Input: part model. Units: mm. Frame: model coordinates. Face numbers are marked on the shaded views. A direction names the side the tool comes from. Give positions to 0.01 mm unless a question says otherwise; leave off trailing zeros. Write each loop counter-clockwise with the first axis right and the second up, starting at its lowest first coordinate (ties: lowest second). Pieces come first, ordered by that corner, then holes. Notation, with made-up numbers: (27.25, -18) - (56.25, -18) arc R30 ccw to (56.25, 5) - close; hole circle Ø8 at (67.25, 6.5). An arc over 180 degrees is marked (long way). Answer as a JSON object with one key per item and string values. Group by question number.
from build123d import *

# Parameters (mm, degrees)
SKETCH_1_R               = 7
EXTRUDE_1_DEPTH          = 12.4
SKETCH_2_W               = 10.589204791
SKETCH_2_H               = 7.5
EXTRUDE_2_DEPTH          = 2
SKETCH_3_R               = 5
CUT_EXTRUDE_1_DEPTH      = 8
CUT_EXTRUDE_1_DEPTH_BACK = 1.5
SKETCH_4_R               = 3.1
CUT_EXTRUDE_2_DEPTH      = 16


with BuildPart() as part:
    # Эскиз1 → Бобышка-Вытянуть1 (new body)
    with BuildSketch(Plane.XY):
        Circle(SKETCH_1_R)
    extrude(amount=EXTRUDE_1_DEPTH)

    # Эскиз2 → Бобышка-Вытянуть2 (add)
    with BuildSketch(Plane.XY):
        with Locations((-11.205397604, 0)):
            Rectangle(SKETCH_2_W, SKETCH_2_H)
    extrude(amount=EXTRUDE_2_DEPTH)

    # Эскиз3 → Вырез-Вытянуть1 (cut, two sides)
    with BuildSketch(Plane(origin=(0, 0, 0), x_dir=(0, 0, -1), z_dir=(1, 0, 0))) as cut_extrude_1_sk:
        with Locations((-6.2, 0)):
            Circle(SKETCH_3_R)
    extrude(amount=CUT_EXTRUDE_1_DEPTH, mode=Mode.SUBTRACT)
    extrude(cut_extrude_1_sk.sketch, amount=-CUT_EXTRUDE_1_DEPTH_BACK, mode=Mode.SUBTRACT)

    # Эскиз4 → Вырез-Вытянуть2 (cut, through all)
    with BuildSketch(Plane(origin=(-1.5, 0, 0), x_dir=(0, 0, -1), z_dir=(1, 0, 0))):
        with Locations((-6.2, 0)):
            Circle(SKETCH_4_R)
    extrude(amount=-CUT_EXTRUDE_2_DEPTH, mode=Mode.SUBTRACT)


solid = part.part
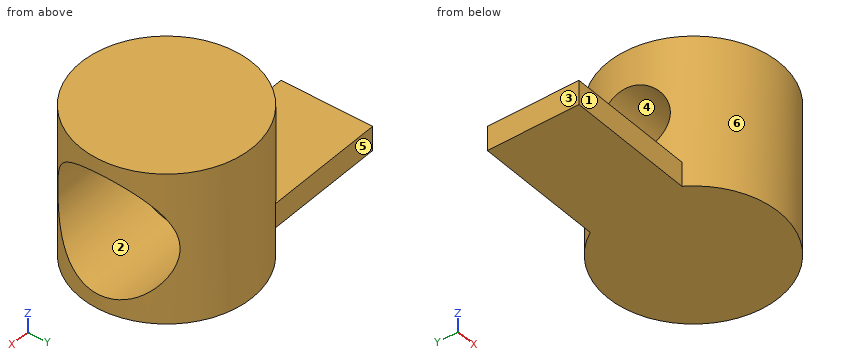
1) Reachability of the marked faces 1, 2 and 3 from +Z, -Z, +X, -X, +Y, -Y: full face, straight path, thin tool, end or side. Return the list, or none.
2) Cut plane A-A on y = 0. Return the cut outline in (x, z), and give its area (3 significant figures).
3) Cut plane C-C on z = 5. Return the cut outline in (x, y).
4) Cut plane D-D on y = 2.75. Return the cut outline in (x, z).
5) Cut plane B-B on x = 0. Return the cut outline in (y, z).
6) Line query: line 1 along Z through (x, y) = (4.75, 0); line 2 along Z through (x, y) = (-5, 0); line 3 along X through (y, z) = (0, 11.75). Output: solid intervals per line, ascending. Write a range as from..to.
7) Mould query, pull axis Y, two halves, no side actions, for the marked faces 4, 5 and 6. Classes: +Y half, -Y half, draft (parallel to the pull), parting line (faces both ways), or undercut.
8) Pin query (flat end, axial travel): P1, Ø6, axis at x = -9, y = 5, coming from the +Z side; P2, Ø1, axis at y = 1, z = 3, coming from the +X side; P3, Ø2, axis at x = -12, z = 0.5, coming from the +Y side. Return the tip coordinate at first contact, or that it passes through.
Filled in:
{
 "1": {"face 1": "+Z, -Z, -X, -Y", "face 2": "+X", "face 3": "+Z, -Z, -X, +Y, -Y"},
 "2": {"outline": "(-16.5, 0) - (7, 0) - (7, 1.2) - (-1.5, 1.2) - (-1.5, 3.1) - (-7, 3.1) - (-7, 2) - (-16.5, 2) - close; (-7, 9.3) - (-1.5, 9.3) - (-1.5, 11.2) - (7, 11.2) - (7, 12.4) - (-7, 12.4) - close", "area": "73.5 mm²"},
 "3": {"outline": "(-6.39, -2.86) arc R7 ccw to (5.04, -4.85) - (-1.5, -4.85) - (-1.5, -2.86) - close; (-6.39, 2.86) - (-1.5, 2.86) - (-1.5, 4.85) - (5.04, 4.85) arc R7 ccw to start"},
 "4": {"outline": "(-16.5, 0) - (6.44, 0) - (6.44, 2.02) - (-1.5, 2.02) - (-1.5, 4.77) - (-6.44, 4.77) - (-6.44, 2) - (-16.5, 2) - close; (-6.44, 7.63) - (-1.5, 7.63) - (-1.5, 10.38) - (6.44, 10.38) - (6.44, 12.4) - (-6.44, 12.4) - close"},
 "5": {"outline": "(-7, 0) - (7, 0) - (7, 12.4) - (-7, 12.4) - close; hole circle Ø10 at (0, 6.2)"},
 "6": {"line 1": "z = 0..1.2, 11.2..12.4", "line 2": "z = 0..3.1, 9.3..12.4", "line 3": "x = -7..7"},
 "7": {"face 4": "undercut", "face 5": "+Y half", "face 6": "parting line"},
 "8": {"P1": "stops at z = 2", "P2": "stops at x = -1.5", "P3": "stops at y = 3.75"}
}
